Autodesk Inventor part; units mm, degrees
ref_plane "YZ Plane" through (0, 0, 0) normal (1, 0, 0) x (0, 1, 0)
ref_plane "XZ Plane" through (0, 0, 0) normal (0, 1, 0) x (-1, 0, 0)
ref_plane "XY Plane" through (0, 0, 0) normal (0, 0, 1) x (1, 0, 0)
sketch "Sketch1" plane through (0, 0, 0) normal (0, 0, 1) x (1, 0, 0)
  line L0 (0, 0) -> (0, 54)
  line L1 (0, 54) -> (55, 54)
  line L2 (55, 54) -> (55, 64)
  line L3 (55, 64) -> (65, 64)
  line L4 (65, 64) -> (65, -6)
  line L5 (65, -6) -> (0, 0)
  line L6 (5, 49) -> (8, 49)
  line L7 (8, 49) -> (8, 41)
  line L8 (8, 41) -> (5, 41)
  line L9 (5, 41) -> (5, 49)
  line L10 (5, 36) -> (8, 36)
  line L11 (8, 36) -> (8, 28)
  line L12 (8, 28) -> (5, 28)
  line L13 (5, 28) -> (5, 36)
  line L14 (5, 23) -> (8, 23)
  line L15 (8, 23) -> (8, 15)
  line L16 (8, 15) -> (5, 15)
  line L17 (5, 15) -> (5, 23)
  line L18 (5, 10) -> (8, 10)
  line L19 (8, 10) -> (8, 2)
  line L20 (8, 2) -> (5, 2)
  line L21 (5, 2) -> (5, 10)
  line L22 (59.5, 54) -> (62.5, 54)
  line L23 (62.5, 54) -> (62.5, 46)
  line L24 (62.5, 46) -> (59.5, 46)
  line L25 (59.5, 46) -> (59.5, 54)
  line L26 (59.5, 41) -> (62.5, 41)
  line L27 (62.5, 41) -> (62.5, 33)
  line L28 (62.5, 33) -> (59.5, 33)
  line L29 (59.5, 33) -> (59.5, 41)
  line L30 (59.5, 28) -> (62.5, 28)
  line L31 (62.5, 28) -> (62.5, 20)
  line L32 (62.5, 20) -> (59.5, 20)
  line L33 (59.5, 20) -> (59.5, 28)
  line L34 (59.5, 15) -> (62.5, 15)
  line L35 (62.5, 15) -> (62.5, 7)
  line L36 (62.5, 7) -> (59.5, 7)
  line L37 (59.5, 7) -> (59.5, 15)
  point P0 (6.5, 49)
  point P1 (6.5, 36)
  point P2 (6.5, 23)
  point P3 (6.5, 10)
  point P4 (6.5, 41)
  point P5 (6.5, 28)
  point P6 (6.5, 15)
  point P7 (5, 6)
  point P8 (61, 54)
  point P9 (61, 41)
  point P10 (61, 28)
  point P11 (61, 15)
  point P12 (61, 46)
  point P13 (61, 33)
  point P14 (61, 20)
  point P15 (59.5, 11)
  point P16 (60, 64)
  point P17 (62.5, 37)
  dimension "d0" = 54
  dimension "d1" = 55
  dimension "d2" = 10
  dimension "d3" = 10
  dimension "d4" = 70
  dimension "d5" = 3
  dimension "d6" = 8
  dimension "d7" = 5
  dimension "d8" = 5
  dimension "d9" = 3
  dimension "d10" = 8
  dimension "d11" = 3
  dimension "d12" = 8
  dimension "d13" = 3
  dimension "d14" = 8
  dimension "d15" = 5
  dimension "d16" = 5
  dimension "d17" = 5
  dimension "d18" = 5
  dimension "d19" = 5
  dimension "d20" = 5
  dimension "d21" = 3
  dimension "d22" = 8
  dimension "d23" = 3
  dimension "d24" = 8
  dimension "d25" = 3
  dimension "d26" = 8
  dimension "d27" = 3
  dimension "d28" = 8
  dimension "d29" = 5
  dimension "d30" = 5
  dimension "d31" = 5
  dimension "d32" = 10
  dimension "d33" = 2.5
  dimension "d34" = 2.5
  dimension "d35" = 2.5
  dimension "d36" = 2.5
extrude "Extrusion1" add sketch "Sketch1" along normal blind 3
properties part number "support select pt 1"
Geometry check sheet. Reference: the model listing, model coordinates, mm. A direction names the side the tool comes from. Coordinates: 2 decimals unless noted, no trailing zeros. Write each loop counter-clockwise with the first axis right and the second up, starting at its lowest first coordinate (ties: lowest second). Pieces come first, ordered by that corner, then holes. Notation, with made-up numbers: M -26,60.25 L 12,60.25 A18 ccw 12,78.25 Z; hole C 32.5,54 d4. An arc over 180 degrees is marked long. Answer as a JSON object with one key per item and string values.
1. Draft check along X on faces 3 (the flat face through (32.95, -3.04, 1.48)), 4 (the flat face through (60, 64, 1)), 5 (the flat face through (62.5, 50, 1)). Enter one of: released by +X, released by -X, zero draft, split by the parting line, or undercut.
Answers below:
{"face 3": "released by -X", "face 4": "zero draft", "face 5": "undercut"}
2. Section check C-C, the plane x = 13. Enter the section's corners in (y, z), plus the area to 3 significant figures.
Answers below:
{"outline": "M -1.2,0 L 54,0 L 54,3 L -1.2,3 Z", "area": "166 mm²"}
3. Section check D-D, the plane z = 1.4. Give the number of separate pieces and of enclosed holes in the cut face, plus the area to 3 significant figures.
Answers below:
{"separate pieces": "1", "enclosed holes": "8", "area": "3,610 mm²"}
4. Scan lines: L1, parallel to X at y = 19, z = 2.8; L2, parallel to X at y = 25, z = 2.45; L3, parallel to X at y = 20.5, z = 1.7. Record each from-to range of solid material in increasing order.
Answers below:
{"L1": "x = 0 to 5, 8 to 65", "L2": "x = 0 to 59.5, 62.5 to 65", "L3": "x = 0 to 5, 8 to 59.5, 62.5 to 65"}
5. Section check B-B, the plane y = 9. Enter the section's corners in (x, z).
Answers below:
{"outline": "M 0,0 L 5,0 L 5,3 L 0,3 Z; M 8,0 L 59.5,0 L 59.5,3 L 8,3 Z; M 62.5,0 L 65,0 L 65,3 L 62.5,3 Z"}
6. Tool access check on faces 1 (the flat face through (6, 23, 1)), 2 (the flat face through (27, 54, 1)). Record the directions out of +Z, -Z, +X, -X, +Y, -Y that give a thin tool (end or side, any length) a straight path to the whole face; none if there is none.
Answers below:
{"face 1": "+Z, -Z", "face 2": "+Z, -Z, -X, +Y"}
7. Section check A-A, the plane y = 38.5. Enter the section's corners in (x, z).
Answers below:
{"outline": "M 0,0 L 59.5,0 L 59.5,3 L 0,3 Z; M 62.5,0 L 65,0 L 65,3 L 62.5,3 Z"}
8. Go/stop test with a flat-tipped pin: pin 1 Ø1.5 at (x, z) = (61.5, 1) entering from -Y. Record where the tip stops, or that it passes through.
Answers below:
{"pin 1": "stops at y = -5.75"}
